from build123d import *

# Parameters (mm, degrees)
SKETCH1_R           = 2.25
BOSS_EXTRUDE1_DEPTH = 16
SKETCH4_W           = 8
SKETCH4_H           = 4
BOSS_EXTRUDE3_DEPTH = 4
CUT_EXTRUDE2_DEPTH  = 6


with BuildPart() as part:
    # Sketch1 → Boss-Extrude1 (new body)
    with BuildSketch(Plane(origin=(0, 0, 0), x_dir=(1, 0, 0), z_dir=(0, 1, 0))):
        Polygon((0, 0), (14.292346673, 0), (14.292346673, 11.238609792), (11.156143946, 17.994963368), (21.835642334, 23.763983363), (25.517809154, 25.875036511), (29.085232636, 28.322878493), (32.990082947, 31.710975059), (34.049112719, 33.434353148), (36.126472393, 37.292437563), (36.843322223, 41.087524896), (35.409622564, 41.762207089), (33.385918935, 38.003772992), (31.21539446, 35.564385481), (28.344844636, 33.594713978), (25.109272652, 32.382219348), (21.002122002, 31.901327051), (18.052032719, 32.863111645), (14.769017999, 35.202837629), (11.063605769, 40.049098317), (7.779911083, 40.049098317), (-3.927764052, 33.33687542), (0, 27.612650649), align=None)
        with Locations((6.23417855, 17.258888852)):
            Circle(SKETCH1_R, mode=Mode.SUBTRACT)
    extrude(amount=BOSS_EXTRUDE1_DEPTH)

    # Sketch4 → Boss-Extrude3 (add)
    with BuildSketch(Plane.ZY):
        with Locations((-4, 8)):
            Rectangle(SKETCH4_W, SKETCH4_H)
    extrude(amount=BOSS_EXTRUDE3_DEPTH)

    # Sketch5 → Cut-Extrude2 (cut)
    with BuildSketch(Plane(origin=(0, 10, 0), x_dir=(1, 0, 0), z_dir=(0, 1, 0))):
        with BuildLine():
            Line((-2, 8), (-2, 4.450866614))
            ThreePointArc((-2, 4.450866614), (-1.853553391, 4.097313224), (-1.5, 3.950866614))
            Line((-1.5, 3.950866614), (-0.5, 3.950866614))
            ThreePointArc((-0.5, 3.950866614), (-0.146446609, 4.097313224), (0, 4.450866614))
            Line((0, 4.450866614), (0, 8))
            Line((0, 8), (-2, 8))
        make_face()
        with BuildLine():
            Line((-4, 2), (-4, 0))
            Line((-4, 0), (-2, 0))
            ThreePointArc((-2, 0), (-3.414213562, 0.585786438), (-4, 2))
        make_face()
    extrude(amount=-CUT_EXTRUDE2_DEPTH, mode=Mode.SUBTRACT)


solid = part.part
For this review, take the finished solid that the model builds, in its own axes (mm). A direction names the side the tool comes from. Give positions to 0.01 mm unless a question says otherwise; leave off trailing zeros. Loops run counter-clockwise (first coordinate to the right, second up) from the corner with the lowest first, then second, coordinate; pieces in that order, holes last.
Item 1: For line 1 along X through (y, z) = (14.25, -38); line 2 along X through (y, z) = (11.5, -38.5); line 3 along Z through (x, y) = (7, 12.75), list the stretches that pass through material, from the lowest coordinate up.
Item 2: Tool access review of faces 4 (the flat face through (12.746, 7.888, -14.569)), 5 (the flat face through (-2, 10, -3)), 6 (the flat face through (29.8, 7.888, -34.593)): name each direction out of +Z, -Z, +X, -X, +Y, -Y from which nothing blocks a thin tool from reaching the whole face with its end or side.
Item 3: Take a section at C-C, the plane z = -3. State the section outline as (x, y) points.
Item 4: Take a section at D-D, the plane y = 3.75. State the section outline as (x, z) points, and give its area (3 significant figures).
Item 5: Insertion check: pin 1 (6 mm diameter, centred on x = 32, z = -25.5, fed in from -Y); pin 2 (2 mm diameter, centred on x = 20.5, y = 5, fed in from +Z); pin 3 (1.6 mm diameter, centred on x = -3, y = 8, fed in from -Z); pin 4 (2.5 mm diameter, centred on x = 9.5, y = 9.5, fed in from -Z). Each pin has a flat end and moves straight along its axis. Give the tip position at first contact, or say it passes through.
Item 6: Draft analysis for pull direction X (two halves, no side actions). For faces 1 (the flat face through (-2, 6, -3)), 2 (the flat face through (-4, 8, -5)), 3 (the flat face through (12.942, 7.888, -37.592)), state which applies: +X half, -X half, draft (parallel to the pull), parting line (faces both ways), or undercut.
Item 7: Take a section at A-A, the plane z = -18.5. State the section outline as (x, y) points.
Calculated:
1. line 1: x = 4.21 to 12.63, 33.38 to 36.26
1. line 2: x = 5.08 to 12.25, 33.65 to 36.35
1. line 3: z = -39.6 to -19.37, -15.14 to 0
2. face 4: +X, +Y, -Y
2. face 5: +Z, -X, +Y
2. face 6: -Z, +Y, -Y
3. outline: (-4, 6) - (0, 6) - (0, 0) - (14.29, 0) - (14.29, 16) - (0, 16) - (0, 10) - (-4, 10) - close
4. outline: (-3.93, -33.34) - (7.78, -40.05) - (11.06, -40.05) - (14.77, -35.2) - (18.05, -32.86) - (21, -31.9) - (25.11, -32.38) - (28.34, -33.59) - (31.22, -35.56) - (33.39, -38) - (35.41, -41.76) - (36.84, -41.09) - (36.13, -37.29) - (34.05, -33.43) - (32.99, -31.71) - (29.09, -28.32) - (25.52, -25.88) - (21.84, -23.76) - (11.16, -17.99) - (14.29, -11.24) - (14.29, 0) - (0, 0) - (0, -27.61) - close; hole circle Ø4.5 at (6.23, -17.26)
4. area: 712 mm2
5. pin 1: passes through
5. pin 2: stops at z = -22.5
5. pin 3: stops at z = -34.33
5. pin 4: stops at z = -40.05
6. face 1: draft
6. face 2: -X half
6. face 3: undercut
7. outline: (0, 0) - (4.36, 0) - (4.36, 16) - (0, 16) - close; (8.11, 0) - (12.09, 0) - (12.09, 16) - (8.11, 16) - close
